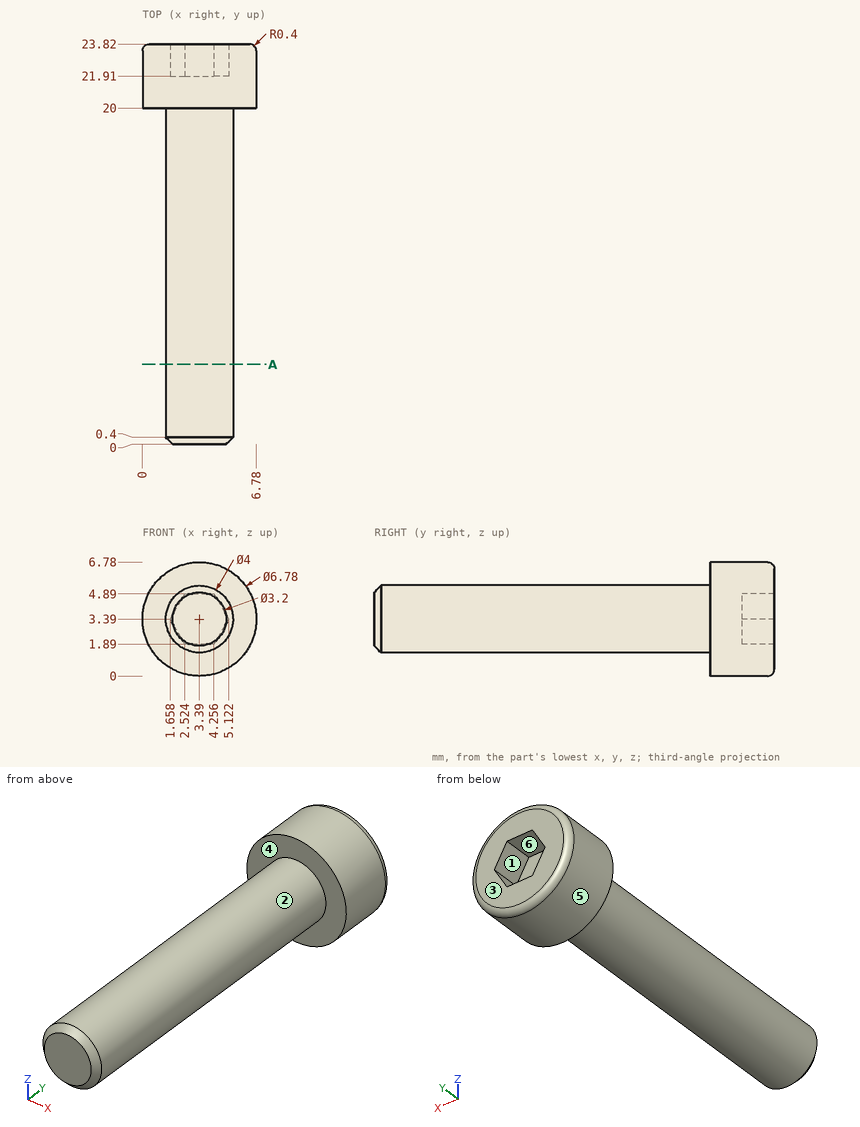
Print and shaded views of the part. All mm, measured from the part's lowest x, y and z. A direction names the side the tool comes from. Round coordinates to 2 decimals unless told otherwise and drop trailing zeros. Order: outer loops, then holes, each group sorted by start corner. A loop starts at its lowest first (then second) coordinate and runs counter-clockwise, first axis right, second up.
Q1. Drop flat-ended pins along their axis: pin 1 (1.5 mm diameter, centred on x = 3.5, y = 13, fed in from -Z); pin 2 (1.5 mm diameter, centred on y = 15.5, z = 5.5, fed in from -X); pin 3 (3 mm diameter, centred on x = 4.5, y = 18, fed in from +Z). Give the stop position or say it passes through.
Q2. Two-plate mould, pull along X, no slides. Class the marked faces 1, 2 and 3: pulls with the +X half, pulls with the -X half, needs draft (parallel to the pull), parting line crosses it, or undercut.
Q3. Wall check: L1, parallel to Z at x = 3.25, y = 22.5; L2, parallel to Z at x = 3.5, y = 10.25; L3, parallel to Y at x = 5.5, z = 4. Give the ranges that are in metal, low to high.
Q4. Slice it at A-A (y = 4.75). Write the cut outline in (x, z).
Q5. Which spindle directions (+Z, -Z, +X, -X, +Y, -Y) get a long thin tool onto all of the face, cutting with end or side? Do the marked faces 4, 5 and 6. Say none if no direction does.
Results below:
1. pin 1: stops at z = 1.39
1. pin 2: stops at x = 1.92
1. pin 3: stops at z = 5.39
2. face 1: undercut
2. face 2: parting line crosses it
2. face 3: needs draft
3. L1: z = 0 to 1.89, 4.89 to 6.78
3. L2: z = 1.39 to 5.39
3. L3: y = 20 to 23.82
4. outline: circle Ø4 at (3.39, 3.39)
5. face 4: -Y
5. face 5: +Y, -Y
5. face 6: +Y
